Here's how the part is built. I have some questions about the finished solid (model axes, mm). A direction names the side the tool comes from. Round coordinates to 2 decimals unless told otherwise and drop trailing zeros. Write each loop counter-clockwise with the first axis right and the second up, starting at its lowest first coordinate (ties: lowest second). Pieces come first, ordered by that corner, then holes. Notation, with made-up numbers: (29, 32) -> (60, 32) arc R5 cw to (60, 38) -> close; hole circle Ø7 at (72.25, 13). An arc over 180 degrees is marked (long way). Answer in a Markdown table with one row per item. Add a question column.
Solid Edge part; units mm, degrees
sketch "Sketch1" plane through (0, 0, 0) normal (0, -1, 0) x (1, 0, 0)
  line L0 (4, 30) -> (4, 0)
  line L1 (4, 0) -> (0, 0)
  line L2 (0, 0) -> (0, 34.4)
  line L3 (0, 34.4) -> (7, 34.4)
  line L4 (7, 34.4) -> (7, 30)
  line L5 (7, 30) -> (4, 30)
revolve "RevolvedProtrusion1" add sketch "Sketch1" angle 360 about axis through (0, 0, 0) along (0, 0, 1)
sketch "Sketch2" plane through (0, 0, 34.4) normal (0, 0, 1) x (1, 0, 0)
  line L0 (1.2028, -2.6242) -> (2.8741, -0.2704)
  line L1 (2.8741, -0.2704) -> (1.6712, 2.3538)
  line L2 (1.6712, 2.3538) -> (-1.2028, 2.6242)
  line L3 (-1.2028, 2.6242) -> (-2.8741, 0.2704)
  line L4 (-2.8741, 0.2704) -> (-1.6712, -2.3538)
  line L5 (-1.6712, -2.3538) -> (1.2028, -2.6242)
extrude "Cutout1" cut sketch "Sketch2" against normal blind 4
cosmetic_thread "Thread1"
chamfer "Chamfer1" distance 0.8 angle 45 8 edges at (0.2342, 2.489, 34.4) (2.0384, -1.4473, 34.4) (-2.2726, -1.0417, 34.4) (-0.2342, -2.489, 34.4) (-2.0384, 1.4473, 34.4) (-4, 0, 0) (2.2726, 1.0417, 34.4) (-7, 0, 30)
fillet "Round1" radius 2.6 1 edges at (-7, 0, 34.4)
properties material "Stainless steel"
Item 1: If we section it at B-B on x = 0: Please give me the cut outline in (y, z).
Item 2: If we section it at A-A on z = 32.5: Please give me the cut outline in (x, y).
Item 3: If we mould it in two halves opening along X, with no side actions, what happens to faces 1 (the flat face through (0.254, 2.487, 32.022)), 2 (the cylindrical face through (-0.867, 3.905, 15.196)), 3 (the flat face through (4, -1.3, 30))? For each: pulls with the +X half, pulls with the -X half, needs draft (parallel to the pull), parting line crosses it, or undercut.
Item 4: On a 3-axis mill with a long thin cutter (end or side, diameter ignored), from which of +Z, -Z, +X, -X, +Y, -Y can I reach the whole of each face in a straight line? I mean faces 4 (the flat face through (2.281, 1.023, 32.022)), 5 (the flat face through (3, -2, 34.4)). Say none if no direction works.
Item 5: I need wall thicknesses on line 1 along Z through (x, y) = (0, 0.25); line 2 along Y through (x, z) = (-1.5, 32); line 3 along X through (y, z) = (-1.25, 19). Which ranges of each line are inside material? Lowest first, please. Write a range as from..to.
Item 6: For P1, Ø3, axis at x = 2, z = 6, coming from the +Y side; P2, Ø6, axis at x = -5.5, y = -2.5, coming from the +Z side; P3, Ø1.5, axis at x = 0, z = 26.5, coming from the -Y side; P4, Ø2.5, axis at x = -1, y = 0.5, coming from the +Z side, each with a flat end and sliding along its axis, tell me the tip position at first contact or that it passes through.
Item 7: If we section it at C-C on z = 10: Please give me the cut outline in (x, y).
Results list:
| question | item | result |
|---|---|---|
| 1 | outline | (-7, 30.8) -> (-6.2, 30) -> (-4, 30) -> (-4, 0.8) -> (-3.2, 0) -> (3.2, 0) -> (4, 0.8) -> (4, 30) -> (6.2, 30) -> (7, 30.8) -> (7, 31.8) arc R2.6 ccw to (4.4, 34.4) -> (3.31, 34.4) -> (2.51, 33.6) -> (2.51, 30.4) -> (-2.51, 30.4) -> (-2.51, 33.6) -> (-3.31, 34.4) -> (-4.4, 34.4) arc R2.6 ccw to (-7, 31.8) -> close |
| 2 | outline | circle Ø13.81 at (0, 0); hole (-2.87, 0.27) -> (-1.67, -2.35) -> (1.2, -2.62) -> (2.87, -0.27) -> (1.67, 2.35) -> (-1.2, 2.62) -> close |
| 3 | face 1 | undercut |
| 3 | face 2 | parting line crosses it |
| 3 | face 3 | needs draft |
| 4 | face 4 | +Z |
| 4 | face 5 | +Z, +X, -X, +Y, -Y |
| 5 | line 1 | 0..30.4 |
| 5 | line 2 | -6.83..-2.37, 2.21..6.83 |
| 5 | line 3 | -3.8..3.8 |
| 6 | P1 | y = 3.97 |
| 6 | P2 | z = 34.4 |
| 6 | P3 | y = -4 |
| 6 | P4 | z = 30.4 |
| 7 | outline | circle Ø8 at (0, 0) |
